Geometry: see drawing. Coordinates: mm, zero at the bounding-box minimum. A direction names the side the tool comes from. Give positions to 0.01 mm unless a question says otherwise; leave off trailing zeros. Write each loop counter-clockwise with the first axis right and the second up, starting at its lowest first coordinate (ties: lowest second). Pieces come first, ordered by that corner, then holes.
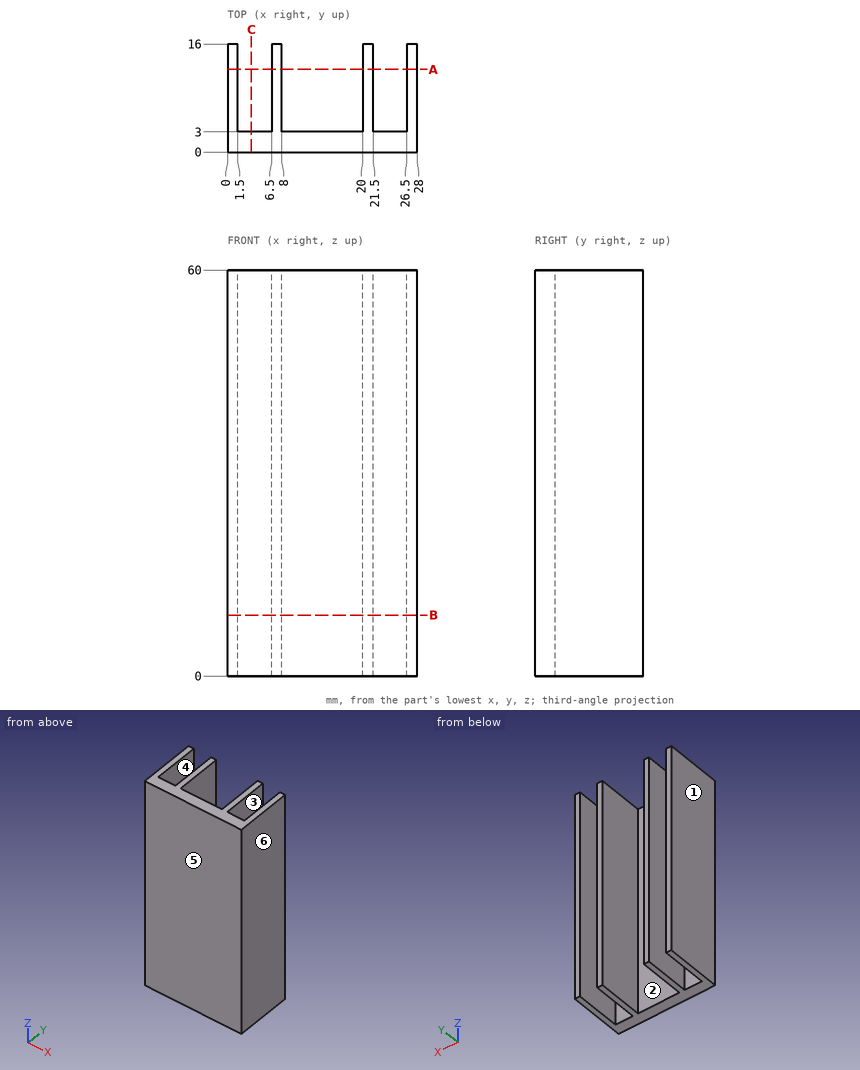
1. Access query for the marked faces 1 and 2. Directions: +Z, -Z, +X, -X, +Y, -Y. A direction counts if a zero-diameter tool reaches every point of the face in a straight line with its end or side. Return the directions, or none.
2. Pin query (flat end, axial travel): P1, Ø1.5, axis at x = 24.5, z = 38, coming from the +Y side. Return the tip coordinate at first contact, or that it passes through.
3. Line query: probe 1 along X at (y, z) = (10.5, 6); probe 2 along Y at (x, z) = (14.75, 27.5). Output: solid intervals per line, ascending.
4. Pull-direction query (X, two-part tool) for the marked faces 3, 4, 5 and 6; classes: pulls with the +X half, pulls with the -X half, needs draft (parallel to the pull), parting line crosses it, or undercut.
5. Section query C-C (x = 3.5). Return loops of the section in (y, z), plus the area to 3 significant figures.
6. Section query B-B (z = 9). Return loops of the section in (x, y).
7. Section query A-A (y = 12.25). Return loops of the section in (x, z), plus the area to 3 significant figures.
The answers:
1. face 1: +Z, -Z, -X, +Y, -Y
1. face 2: +Z, -Z, +Y
2. P1: stops at y = 3
3. probe 1: x = 0 to 1.5, 6.5 to 8, 20 to 21.5, 26.5 to 28
3. probe 2: y = 0 to 3
4. face 3: undercut
4. face 4: undercut
4. face 5: needs draft
4. face 6: pulls with the +X half
5. outline: (0, 0) - (3, 0) - (3, 60) - (0, 60) - close
5. area: 180 mm2
6. outline: (0, 0) - (28, 0) - (28, 16) - (26.5, 16) - (26.5, 3) - (21.5, 3) - (21.5, 16) - (20, 16) - (20, 3) - (8, 3) - (8, 16) - (6.5, 16) - (6.5, 3) - (1.5, 3) - (1.5, 16) - (0, 16) - close
7. outline: (0, 0) - (1.5, 0) - (1.5, 60) - (0, 60) - close; (6.5, 0) - (8, 0) - (8, 60) - (6.5, 60) - close; (20, 0) - (21.5, 0) - (21.5, 60) - (20, 60) - close; (26.5, 0) - (28, 0) - (28, 60) - (26.5, 60) - close
7. area: 360 mm2
